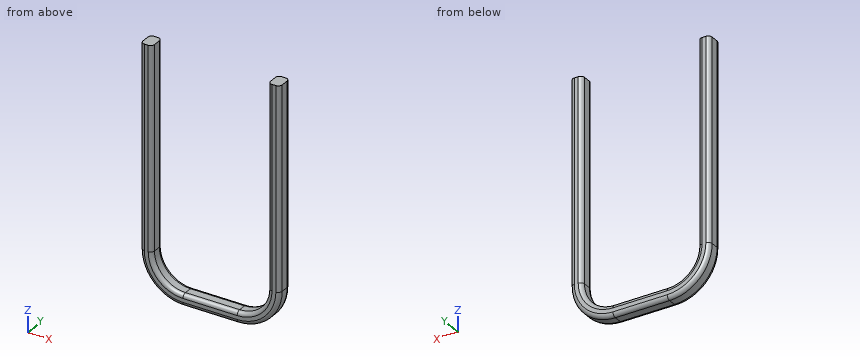
from build123d import *

# Parameters (mm, degrees)
SKETCH2_W = 0.75
SKETCH2_H = 1
FILLET1_R = 0.25


with BuildPart() as part:
    # Sweep1: sweep along a path in Sketch1
    with BuildLine(Plane(origin=(0, 0, 0), x_dir=(1, 0, 0), z_dir=(0, 1, 0))) as sweep1_path:
        Line((-3.95, 0), (-3.95, 13))
        ThreePointArc((-3.95, 13), (-3.364213562, 14.414213562), (-1.95, 15))
        Line((-1.95, 15), (1.553078387, 15))
        ThreePointArc((1.553078387, 15), (2.96729195, 14.414213562), (3.553078387, 13))
        Line((3.553078387, 13), (3.553078387, 0))
    # Sketch2 → Sweep1 (sweep)
    with BuildSketch(Plane.XY):
        with Locations((-4.325, 0.5)):
            Rectangle(SKETCH2_W, SKETCH2_H)
    sweep(path=sweep1_path.line)

    # Fillet1
    fillet1_edges = [part.edges().sort_by_distance(p)[0] for p in [
        (-3.364213562, 1, -14.414213562),
        (-3.894543648, 1, -14.944543648),
        (-3.894543648, 0, -14.944543648),
        (-3.364213562, 0, -14.414213562),
        (-0.198460806, 1, -15),
        (-0.198460806, 1, -15.75),
        (-0.198460806, 0, -15.75),
        (-0.198460806, 0, -15),
        (2.96729195, 1, -14.414213562),
        (3.497622036, 1, -14.944543648),
        (3.497622036, 0, -14.944543648),
        (2.96729195, 0, -14.414213562),
        (3.553078387, 1, -6.5),
        (4.303078387, 1, -6.5),
        (4.303078387, 0, -6.5),
        (3.553078387, 0, -6.5),
        (-3.95, 0, -6.5),
        (-4.7, 0, -6.5),
        (-4.7, 1, -6.5),
        (-3.95, 1, -6.5),
    ]]
    fillet(fillet1_edges, radius=FILLET1_R)


solid = part.part
Part model, mm, in its own coordinate system. Give positions to 0.01 mm unless a question says otherwise; leave off trailing zeros. Write each loop counter-clockwise with the first axis right and the second up, starting at its lowest first coordinate (ties: lowest second). Pieces come first, ordered by that corner, then holes.
1) Probe L1, parallel to X at y = 0.7, z = -8; L2, parallel to X at y = 0.9, z = -14; L3, parallel to Z at x = 1, y = 0.3. List the from-to ranges inside material, lowest first.
Resolved:
L1: x = -4.7 to -3.95, 3.55 to 4.3
L2: x = -4.46 to -3.74, 3.34 to 4.06
L3: z = -15.75 to -15
2) Cut at C-C on x = -1.75. Write the cut outline in (y, z), then the cut area to 3 significant figures.
Resolved:
outline: (0, -15.5) arc R0.25 ccw to (0.25, -15.75) - (0.75, -15.75) arc R0.25 ccw to (1, -15.5) - (1, -15.25) arc R0.25 ccw to (0.75, -15) - (0.25, -15) arc R0.25 ccw to (0, -15.25) - close
area: 0.696 mm2
3) Pin check, flat tip, straight feed: pin 1 (1 mm diameter, centred on x = 2.5, z = -2, fed in from -Y). Stop position of the tip, or through.
Resolved:
pin 1: passes through
4) Cut at B-B on y = 0.45. Write the cut outline in (x, z), then the cut area to 3 significant figures.
Resolved:
outline: (-4.7, -13) arc R2.75 ccw to (-1.95, -15.75) - (1.55, -15.75) arc R2.75 ccw to (4.3, -13) - (4.3, 0) - (3.55, 0) - (3.55, -13) arc R2 cw to (1.55, -15) - (-1.95, -15) arc R2 cw to (-3.95, -13) - (-3.95, 0) - (-4.7, 0) - close
area: 27.7 mm2
5) Cut at A-A on z = -7. Write the cut outline in (x, y), then the cut area to 3 significant figures.
Resolved:
outline: (-4.7, 0.25) arc R0.25 ccw to (-4.45, 0) - (-4.2, 0) arc R0.25 ccw to (-3.95, 0.25) - (-3.95, 0.75) arc R0.25 ccw to (-4.2, 1) - (-4.45, 1) arc R0.25 ccw to (-4.7, 0.75) - close; (3.55, 0.25) arc R0.25 ccw to (3.8, 0) - (4.05, 0) arc R0.25 ccw to (4.3, 0.25) - (4.3, 0.75) arc R0.25 ccw to (4.05, 1) - (3.8, 1) arc R0.25 ccw to (3.55, 0.75) - close
area: 1.39 mm2
